```python
from build123d import *

# Parameters (mm, degrees)
FILLET1_R      = 0.5
RIB1_REACH     = 43.569
SKETCH2_WALL_W = 87.966865888
SKETCH2_WALL_H = 2


with BuildPart() as part:
    # Sketch1 → Revolve1 (revolve)
    with BuildSketch(Plane.XY, mode=Mode.PRIVATE) as revolve1_sk:
        Polygon((0, 8), (0, 0), (40, 0), (40, 3.75), (37.73, 3.75), (37.73, 3.2), (37, 3.2), (37, 3.75), (2, 3.75), (2, 8), align=None)
    revolve(revolve1_sk.sketch.rotate(Axis((0, 0, 0), (1, 0, 0)), 90), axis=Axis((0, 0, 0), (1, 0, 0)))

    # Fillet1
    fillet1_edges = [part.edges().sort_by_distance(p)[0] for p in [
        (0, 0, -8),
        (2, 0, -8),
    ]]
    fillet(fillet1_edges, radius=FILLET1_R)

    # Sketch2 wall → Rib1 (add, up to next)
    with BuildSketch(Plane(origin=(3, 4.75, 0), x_dir=(-0.707106781187, 0.707106781187, 0), z_dir=(-0.707106781187, -0.707106781187, 0)), mode=Mode.PRIVATE) as rib1_sk1:
        Rectangle(SKETCH2_WALL_W, SKETCH2_WALL_H)
    rib1_tool1 = extrude(rib1_sk1.sketch, amount=RIB1_REACH, mode=Mode.PRIVATE) - part.part
    add(rib1_tool1.solids().sort_by_distance((3, 4.75, 0))[0])


solid = part.part
```
Can you work these out from the model? Positions are in its coordinate system, mm. A direction names the side the tool comes from. Coordinates: 2 decimals unless noted, no trailing zeros. Loops run counter-clockwise (first coordinate to the right, second up) from the corner with the lowest first, then second, coordinate; pieces in that order, holes last.
1) Imagine slicing it at A-A on y = 0. List the corners of the cut face in (x, z) for me, plus the area to 3 significant figures.
2) I need wall thicknesses on probe 1 along X at (y, z) = (-6.25, 3.25); probe 2 along Y at (x, z) = (12.5, 0); probe 3 along Z at (x, y) = (18, -2.75). Which ranges of each line are inside material? Lowest first, please.
3) Thinking about a two-plate mould opening in X: for faces 5 (the flat face through (0, 0, 0)), 6 (the cylindrical face through (37.36, -0.961, 3.052)), 7 (the flat face through (2, 3, -3)), which applies, pulls with the +X half, pulls with the -X half, needs draft (parallel to the pull), parting line crosses it, or undercut?
4) For pin 1 (0.6 mm diameter, centred on x = 3, y = 4.5, fed in from -Z); pin 2 (0.6 mm diameter, centred on x = 2.5, y = 5, fed in from +Z); pin 3 (6 mm diameter, centred on x = 33.5, y = -3.5, fed in from +Z); pin 4 (4 mm diameter, centred on x = 10, y = -6.5, fed in from +Z), each with a flat end and sliding along its axis, tell me the tip position at first contact or that it passes through.
5) Imagine slicing it at B-B on z = 0. List the corners of the cut face in (x, y) for me, plus the area to 3 significant figures.
6) Imagine slicing it at C-C on x = 34. List the corners of the cut face in (y, z) for me, plus the area to 3 significant figures.
7) Which directions (+Z, -Z, +X, -X, +Y, -Y) give clear straight access to the entire face, cutting with the end or side of a thin tool? Please do faces 1 (the cylindrical face through (38.85, -3.16, 2.02)), 2 (the flat face through (3, 4, -1)), 3 (the flat face through (40, 0, 0)), 4 (the flat face through (3, 4, 1)).
Completed:
1. outline: (0, -7.5) arc R0.5 ccw to (0.5, -8) - (1.5, -8) arc R0.5 ccw to (2, -7.5) - (2, -3.75) - (37, -3.75) - (37, -3.2) - (37.73, -3.2) - (37.73, -3.75) - (40, -3.75) - (40, 3.75) - (37.73, 3.75) - (37.73, 3.2) - (37, 3.2) - (37, 3.75) - (2, 3.75) - (2, 7.5) arc R0.5 ccw to (1.5, 8) - (0.5, 8) arc R0.5 ccw to (0, 7.5) - close
1. area: 316 mm2
2. probe 1: x = 0 to 2
2. probe 2: y = -3.75 to 3.75
2. probe 3: z = -2.55 to 2.55
3. face 5: pulls with the -X half
3. face 6: undercut
3. face 7: pulls with the +X half
4. pin 1: stops at z = -1
4. pin 2: stops at z = 1
4. pin 3: stops at z = 3.72
4. pin 4: passes through
5. outline: (0, -7.5) arc R0.5 ccw to (0.5, -8) - (1.5, -8) arc R0.5 ccw to (2, -7.5) - (2, -3.75) - (37, -3.75) - (37, -3.2) - (37.73, -3.2) - (37.73, -3.75) - (40, -3.75) - (40, 3.75) - (37.73, 3.75) - (37.73, 3.2) - (37, 3.2) - (37, 3.75) - (4, 3.75) - (2, 5.75) - (2, 7.5) arc R0.5 ccw to (1.5, 8) - (0.5, 8) arc R0.5 ccw to (0, 7.5) - close
5. area: 318 mm2
6. outline: circle Ø7.5 at (0, 0)
6. area: 44.2 mm2
7. face 1: +X
7. face 2: -Z, +X, +Y
7. face 3: +Z, -Z, +X, +Y, -Y
7. face 4: +Z, +X, +Y
